```python
from build123d import *

# Parameters (mm, degrees)
SKETCH14_W         = 99.852899645
SKETCH14_H         = 2
CUT_EXTRUDE1_DEPTH = 50


with BuildPart() as part:
    # Sketch1 → Revolve1 (revolve)
    with BuildSketch(Plane(origin=(0, 0, 0), x_dir=(-1, 0, 0), z_dir=(0, 0, -1)), mode=Mode.PRIVATE) as revolve1_sk:
        with BuildLine():
            Line((-763.382394472, 85), (-763.235294117, 85))
            ThreePointArc((-763.235294117, 85), (-380.825050597, 49.616912867), (0, 0))
            Line((0, 0), (18.46847438, 0))
            Line((18.46847438, 0), (0.295326728, 1.978075358))
            ThreePointArc((0.295326728, 1.978075358), (-380.640283603, 51.608700281), (-763.161647781, 87))
            Line((-763.161647781, 87), (-763.382394472, 87))
            Line((-763.382394472, 87), (-763.382394472, 85))
        make_face()
    revolve(revolve1_sk.sketch.rotate(Axis((763.235294117, 0, 0), (-1, 0, 0)), 180), axis=Axis((763.235294117, 0, 0), (-1, 0, 0)))

    # Sketch14 → Revolve4 (revolve)
    with BuildSketch(Plane(origin=(0, 0, 0), x_dir=(-1, 0, 0), z_dir=(0, 0, -1)), mode=Mode.PRIVATE) as revolve4_sk:
        with Locations((-813.308844295, 86)):
            Rectangle(SKETCH14_W, SKETCH14_H)
    revolve(revolve4_sk.sketch.rotate(Axis((763.235294117, 0, 0), (1, 0, 0)), 180), axis=Axis((763.235294117, 0, 0), (1, 0, 0)))

    # Sketch15 → Cut-Extrude1 (cut, symmetric)
    with BuildSketch(Plane.XY):
        Polygon((-1798.394426372, -1.080422086), (-17.779665104, -0.07497417), (114.997091286, 0), (114.997091286, 42.308767364), (-24.793740749, 42.308767364), (-24.793740749, -36.098631976), (114.997091286, -36.098631976), (114.997091286, 0), (114.997091286, 1780.615045137), (-2311.882223875, 4386.879909942), (-4225.273741533, 2605.184442719), align=None)
    extrude(amount=CUT_EXTRUDE1_DEPTH, both=True, mode=Mode.SUBTRACT)


with BuildPart() as cut_extrude1_kept_piece:
    # of the separate pieces the step leaves, the one the design keeps (cut_extrude1_pieces_kept)
    add(part.part.solids().sort_by_distance((763.161647781, -87, 0))[0])


solid = cut_extrude1_kept_piece.part
```
Input: part model. Units: mm. Frame: model coordinates. Give positions to 0.01 mm unless a question says otherwise; leave off trailing zeros. Order: outer loops, then holes, each group sorted by start corner. A loop starts at its lowest first (then second) coordinate and runs counter-clockwise, first axis right, second up.
1. Cut plane A-A (x = 790). Return loops of the section in (y, z), and give its area (3 significant figures).
Computed:
outline: circle Ø174 at (0, 0); hole circle Ø170 at (0, 0)
area: 1,080 mm2
2. Line query: probe 1 along Y at (x, z) = (763, 0); probe 2 along Z at (x, y) = (386.5, 39.5). Output: solid intervals per line, ascending.
Computed:
probe 1: y = -86.99 to -84.98, 84.98 to 86.99
probe 2: z = -34.22 to -31.06, 31.06 to 34.22
3. Pin query (flat end, axial travel): pin 1 Ø3 at (x, y) = (461, 32.5) entering from +Z; pin 2 Ø1 at (x, y) = (464.5, -17.5) entering from -Z; pin 3 Ø5 at (x, z) = (746.5, -20.5) entering from +Y. Return the tip coordinate at first contact, or that it passes through.
Computed:
pin 1: stops at z = 51.67
pin 2: stops at z = -58.18
pin 3: stops at y = 83.88
